The model under review builds one solid part; all positions refer to its coordinate system, in mm. A direction names the side the tool comes from. Round coordinates to 2 decimals unless told otherwise and drop trailing zeros. Order: outer loops, then holes, each group sorted by start corner. A loop starts at its lowest first (then second) coordinate and runs counter-clockwise, first axis right, second up. Notation, with made-up numbers: M -1.5,-2 L 47.5,-2 A17 cw 47.5,2 Z; hole C 1.5,19.25 d3. An arc over 180 degrees is marked long. One line per item, written item: value. Start each with the question number.
from build123d import *

# Parameters (mm, degrees)
SKIZZE1_R                            = 10.65
SKIZZE1_R_2                          = 8
AUFSATZ_LINEAR_AUSTRAGEN1_DEPTH      = 100
SKIZZE2_W                            = 10
SKIZZE2_H                            = 5
SCHNITT_LINEAR_AUSTRAGEN1_DEPTH      = 10
SCHNITT_LINEAR_AUSTRAGEN1_DEPTH_BACK = 10


with BuildPart() as part:
    # Skizze1 → Aufsatz-Linear austragen1 (new body)
    with BuildSketch(Plane.XY):
        Circle(SKIZZE1_R)
        Circle(SKIZZE1_R_2, mode=Mode.SUBTRACT)
    extrude(amount=AUFSATZ_LINEAR_AUSTRAGEN1_DEPTH)

    # Skizze2 → Schnitt-Linear austragen1 (cut, two sides)
    with BuildSketch(Plane(origin=(0, 0, 0), x_dir=(0, 0, -1), z_dir=(1, 0, 0))) as schnitt_linear_austragen1_sk:
        with Locations((-30, 8.15)):
            Rectangle(SKIZZE2_W, SKIZZE2_H)
    extrude(amount=SCHNITT_LINEAR_AUSTRAGEN1_DEPTH, mode=Mode.SUBTRACT)
    extrude(schnitt_linear_austragen1_sk.sketch, amount=-SCHNITT_LINEAR_AUSTRAGEN1_DEPTH_BACK, mode=Mode.SUBTRACT)


solid = part.part
Item 1: Clearance check with flat-ended pins moving along their axes: P1, Ø3, axis at x = -2.5, z = 32.5, coming from the -Y side; P2, Ø1, axis at x = -1, z = 63, coming from the +Y side; P3, Ø1, axis at x = 8, z = 29.5, coming from the +Y side. State where each tip first meets the part, or that it passes through.
Item 2: Consider section D-D, the plane y = -4.5. Give the boundary of the cut face in (x, z), then the cut area to 3 significant figures.
Item 3: Wall thickness on L1, parallel to Y at x = 0, z = 67; L2, parallel to X at y = -0.5, z = 77.5; L3, parallel to Y at x = 2.25, z = 60.5: over which ranges is each line inside the solid? List them lowest first.
Item 4: Machinability: for faces 1 (the flat face through (2, 8, 0)), 2 (the flat face through (0, 9, 25)), which of the approach directions +Z, -Z, +X, -X, +Y, -Y give a long, thin tool a straight path to every point of the face, cutting with its end or side? Answer none if there is none.
Item 5: Consider section B-B, the plane y = 0. Give the boundary of the cut face in (x, z), then the cut area to 3 significant figures.
Item 6: The part is to be moulded in two halves that separate along Y. For faces 3 (the flat face through (-7, 5.65, 30)), 4 (the flat face through (0, 9, 35)), 5 (the cylindrical face through (-1.73, -7.81, 49.3)), say which applies: pulls with the +Y half, pulls with the -Y half, needs draft (parallel to the pull), parting line crosses it, or undercut.
Item 7: Consider section C-C, the plane z = 15.5. Give the boundary of the cut face in (x, y), then the cut area to 3 significant figures.
Item 8: Consider section A-A, the plane x = 0. Give the boundary of the cut face in (y, z).
Computed:
1. P1: stops at y = -10.6
1. P2: stops at y = 10.64
1. P3: stops at y = 5.65
2. outline: M -9.65,0 L -6.61,0 L -6.61,100 L -9.65,100 Z; M 6.61,0 L 9.65,0 L 9.65,100 L 6.61,100 Z
2. area: 608 mm^2
3. L1: y = -10.65 to -8, 8 to 10.65
3. L2: x = -10.64 to -7.98, 7.98 to 10.64
3. L3: y = -10.41 to -7.68, 7.68 to 10.41
4. face 1: -Z, +X, -X, +Y, -Y
4. face 2: +X, -X, +Y
5. outline: M -10.65,0 L -8,0 L -8,100 L -10.65,100 Z; M 8,0 L 10.65,0 L 10.65,100 L 8,100 Z
5. area: 530 mm^2
6. face 3: pulls with the +Y half
6. face 4: needs draft
6. face 5: undercut
7. outline: C 0,0 d21.3; hole C 0,0 d16
7. area: 155 mm^2
8. outline: M -10.65,0 L -8,0 L -8,100 L -10.65,100 Z; M 8,0 L 10.65,0 L 10.65,25 L 8,25 Z; M 8,35 L 10.65,35 L 10.65,100 L 8,100 Z
